Build history of the part. All positions in model axes, mm. A direction names the side the tool comes from. Coordinates: 2 decimals unless noted, no trailing zeros. Order: outer loops, then holes, each group sorted by start corner. A loop starts at its lowest first (then second) coordinate and runs counter-clockwise, first axis right, second up. Notation, with made-up numbers: (23.5, 45.5) - (37.5, 45.5) arc R16 cw to (37.5, 63.5) - close; hole circle Ø7 at (51, -18). An arc over 180 degrees is marked (long way). Write each question's results on one line, items separated by ' | '.
from build123d import *

# Parameters (mm, degrees)
F0_W        = 47.4317967892
F0_H        = 20
F0_R        = 4.5
F1_DEPTH    = 15
F2_R        = 7.05
F3_DEPTH    = 25
F7_DEPTH    = 13.25
F8_T1_DEPTH = 20
F0_R_2      = 2.5
F9_DEPTH    = 15


# Not quite as in the source:
# - a fillet or chamfer that OpenCascade refuses, or shapes differently, is made with other operations: its cross-section is extruded or revolved along the edge and cut away or added


with BuildPart() as f1:
    # F0 (on Front) → F1 (new body)
    with BuildSketch(Plane.XZ):
        Rectangle(F0_W, F0_H)
        with Locations((-18.2158983946, 0)):
            Circle(F0_R, mode=Mode.SUBTRACT)
        with Locations((18.2158983946, 0)):
            Circle(F0_R, mode=Mode.SUBTRACT)
    extrude(amount=F1_DEPTH)

    # F2 (on face) → F3 (cut)
    with BuildSketch(Plane.XY.offset(10)):
        with Locations((0, -15)):
            Circle(F2_R)
    extrude(amount=-F3_DEPTH, mode=Mode.SUBTRACT)

    # F4 (on face) → F5 (revolve, cut)
    with BuildSketch(Plane.XZ.offset(15)):
        with BuildLine():
            Line((-7.05, -10), (-7.05, 10))
            ThreePointArc((-7.05, 10), (-12.2352972992, 0), (-7.05, -10))
        make_face()
    revolve(axis=Axis((0, -15, 0.0368109904), (0, 0, -1)), mode=Mode.SUBTRACT)

    # F6 (on face) → F7 (cut)
    with BuildSketch(Plane.XZ.offset(15)):
        Polygon((2.5, -10.0813228637), (2.5, 10), (0, 10), (-2.5, 10), (-2.5, -10.0813228637), (0, -10.0813228637), align=None)
    extrude(amount=-F7_DEPTH, mode=Mode.SUBTRACT)

    # F8: fillet of radius 1 on 2 edges, made by hand

    # F8_s2 → F8_t1 (join)
    with BuildSketch(Plane.XY.offset(-10)):
        with BuildLine():
            add(Edge.make_bspline(
                [(1.5, -1.75), (2.5, -1.75), (2.5, -2.75)],
                knots=[0, 0, 0, 1, 1, 1], degree=2, weights=[1, 2.3333333333, 1]))
            Line((2.5, -2.75), (2.5, -1.75))
            Line((2.5, -1.75), (1.5, -1.75))
        make_face()
        with BuildLine():
            add(Edge.make_bspline(
                [(-2.5, -2.75), (-2.5, -1.75), (-1.5, -1.75)],
                knots=[0, 0, 0, 1, 1, 1], degree=2, weights=[1, 2.3333333333, 1]))
            Line((-1.5, -1.75), (-2.5, -1.75))
            Line((-2.5, -1.75), (-2.5, -2.75))
        make_face()
    extrude(amount=F8_T1_DEPTH)

    # F0 (on Front) → F9 (join)
    with BuildSketch(Plane.XZ):
        with Locations((-18.2158983946, 0)):
            Circle(F0_R)
        with Locations((-18.2158983946, 0)):
            Circle(F0_R_2, mode=Mode.SUBTRACT)
        with Locations((18.2158983946, 0)):
            Circle(F0_R)
        with Locations((18.2158983946, 0)):
            Circle(F0_R_2, mode=Mode.SUBTRACT)
    extrude(amount=F9_DEPTH)


solid = f1.part
1. Band-saw the part on A-A on z = 0. Give the number of separate pieces and of enclosed holes in the cut face, then the cut area to 3 significant figures.
Solved:
separate pieces: 3 | enclosed holes: 0 | area: 321 mm2
2. Probe line 1 (Z direction, x = 18, y = -6.5); line 2 (X direction, y = -6.5, z = -2); line 3 (X direction, y = -10.5, z = -7.25). List the from-to ranges inside material, lowest first.
Solved:
line 1: z = -10 to -2.49, 2.49 to 10 | line 2: x = -23.72 to -19.72, -16.72 to -8.57, 8.57 to 16.72, 19.72 to 23.72 | line 3: x = -23.72 to -8.77, 8.77 to 23.72
3. Band-saw the part on B-B on x = -9. Give the cut face in (y, z).
Solved:
outline: (-15, -10) - (0, -10) - (0, 10) - (-15, 10) - (-15, 8.29) arc R8.29 cw to (-15, -8.29) - close
4. Tool access for faces 4 (the face through (23.716, -7, 0)), 5 (the face through (-2.5, -3, 2)): list every direction of +Z, -Z, +X, -X, +Y, -Y with a clear straight run to the whole face (end or side of a thin tool).
Solved:
face 4: +Z, -Z, +X, +Y, -Y | face 5: +Z, -Z, -Y
5. Two-plate mould, pull along Z, no slides. Class faces 1 (the face through (-6, -7, 10)), 2 (the face through (-15, -15, 0)), 3 (the face through (20.6, -7.4, 0.75)): +Z half, -Z half, draft (parallel to the pull), parting line (faces both ways), or undercut.
Solved:
face 1: +Z half | face 2: draft | face 3: undercut
6. Drop flat-ended pins along their axis: pin 1 Ø8 at (x, z) = (-18.22, 0) entering from +Y; pin 2 Ø3.5 at (x, z) = (-0.5, 4) entering from -Y. Give the stop position or say it passes through.
Solved:
pin 1: stops at y = 0 | pin 2: stops at y = -1.83
